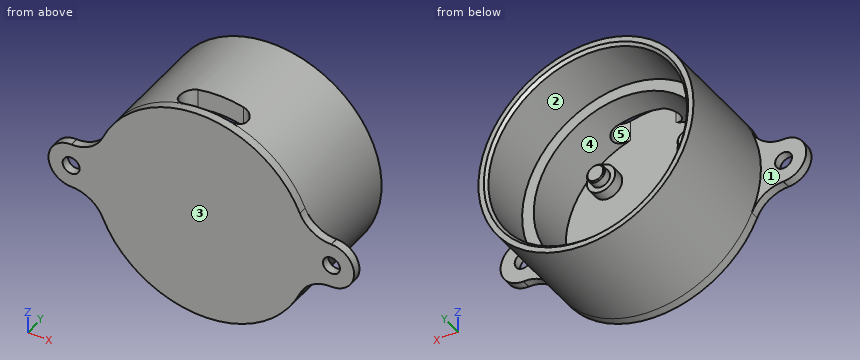
```python
from build123d import *

# Parameters (mm, degrees)
SKETCH_2_R               = 1.5
EXTRUDE_2_DEPTH          = 1.5
SKETCH_3_R               = 19
SKETCH_3_R_2             = 15.5
EXTRUDE_3_DEPTH          = 9
SKETCH_4_R               = 2.5
EXTRUDE_4_DEPTH          = 2
SKETCH_8_R               = 19
SKETCH_8_R_2             = 17.55
EXTRUDE_5_DEPTH          = 10
SKETCH_9_R               = 1.7
SKETCH_9_R_2             = 1.6
EXTRUDE_6_DEPTH          = 1.6
CUT_EXTRUDE_2_REACH      = 53.674
CUT_EXTRUDE_2_END_RADIUS = 15.5
CHAMFER_1_SIZE           = 0.5
CHAMFER_2_SIZE           = 0.2


with BuildPart() as part:
    # Эскиз2 → Бобышка-Вытянуть2 (new body)
    with BuildSketch(Plane(origin=(0, 0, 0), x_dir=(1, 0, 0), z_dir=(0, 1, 0))):
        with BuildLine():
            Line((-23, 4), (-22.912878475, 4))
            ThreePointArc((-22.912878475, 4), (-19.62654313, 4.980039841), (-17.413787641, 7.6))
            ThreePointArc((-17.413787641, 7.6), (0, 19), (17.413787641, 7.6))
            ThreePointArc((17.413787641, 7.6), (19.62654313, 4.980039841), (22.912878475, 4))
            Line((22.912878475, 4), (23, 4))
            ThreePointArc((23, 4), (27, 0), (23, -4))
            Line((23, -4), (22.912878475, -4))
            ThreePointArc((22.912878475, -4), (19.62654313, -4.980039841), (17.413787641, -7.6))
            ThreePointArc((17.413787641, -7.6), (0, -19), (-17.413787641, -7.6))
            ThreePointArc((-17.413787641, -7.6), (-19.62654313, -4.980039841), (-22.912878475, -4))
            Line((-22.912878475, -4), (-23, -4))
            ThreePointArc((-23, -4), (-27, 0), (-23, 4))
        make_face()
        with Locations(Location((-23, 0, 0), (0, 0, 270))):
            Circle(SKETCH_2_R, mode=Mode.SUBTRACT)
        with Locations(Location((23, 0, 0), (0, 0, 90))):
            Circle(SKETCH_2_R, mode=Mode.SUBTRACT)
    extrude(amount=EXTRUDE_2_DEPTH)

    # Эскиз3 → Бобышка-Вытянуть3 (add)
    with BuildSketch(Plane(origin=(0, 1.5, 0), x_dir=(1, 0, 0), z_dir=(0, 1, 0))):
        with Locations(Location((0, 0, 0), (0, 0, 23.578178478))):
            Circle(SKETCH_3_R)
        with Locations(Location((0, 0, 0), (0, 0, 270))):
            Circle(SKETCH_3_R_2, mode=Mode.SUBTRACT)
    extrude(amount=EXTRUDE_3_DEPTH)

    # Эскиз4 → Бобышка-Вытянуть4 (add)
    with BuildSketch(Plane(origin=(0, 1.5, 0), x_dir=(1, 0, 0), z_dir=(0, 1, 0))):
        with Locations(Location((-8, -8, 0), (0, 0, 90))):
            Circle(SKETCH_4_R)
        with Locations(Location((8, -8, 0), (0, 0, 90))):
            Circle(SKETCH_4_R)
        with Locations(Location((8, 8, 0), (0, 0, 90))):
            Circle(SKETCH_4_R)
        with Locations(Location((-8, 8, 0), (0, 0, 90))):
            Circle(SKETCH_4_R)
    extrude(amount=EXTRUDE_4_DEPTH)

    # Эскиз8 → Бобышка-Вытянуть5 (add)
    with BuildSketch(Plane(origin=(0, 10.5, 0), x_dir=(1, 0, 0), z_dir=(0, 1, 0))):
        with Locations(Location((0, 0, 0), (0, 0, 23.578178478))):
            Circle(SKETCH_8_R)
        with Locations(Location((0, 0, 0), (0, 0, 270))):
            Circle(SKETCH_8_R_2, mode=Mode.SUBTRACT)
    extrude(amount=EXTRUDE_5_DEPTH)

    # Эскиз9 → Бобышка-Вытянуть6 (add)
    with BuildSketch(Plane(origin=(0, 3.5, 0), x_dir=(1, 0, 0), z_dir=(0, 1, 0))):
        with Locations(Location((-8, 8, 0), (0, 0, 270))):
            Circle(SKETCH_9_R)
        with Locations(Location((8, 8, 0), (0, 0, 270))):
            Circle(SKETCH_9_R_2)
        with Locations(Location((-8, -8, 0), (0, 0, 270))):
            Circle(SKETCH_9_R_2)
        with Locations(Location((8, -8, 0), (0, 0, 270))):
            Circle(SKETCH_9_R_2)
    extrude(amount=EXTRUDE_6_DEPTH)

    # Вырез-Вытянуть2: up to this cylinder (the profile starts outside it)
    cut_extrude_2_end = Plane(origin=(0, 3.5, 0), z_dir=(0, -1, 0)) * Cylinder(CUT_EXTRUDE_2_END_RADIUS, 139.348, mode=Mode.PRIVATE)
    # Эскиз11 → Вырез-Вытянуть2 (cut, up to the surface)
    with BuildSketch(Plane.XY.offset(20), mode=Mode.PRIVATE) as cut_extrude_2_sk1:
        with BuildLine():
            Line((-4, 5.5), (4, 5.5))
            ThreePointArc((4, 5.5), (6, 3.5), (4, 1.5))
            Line((4, 1.5), (-4, 1.5))
            ThreePointArc((-4, 1.5), (-6, 3.5), (-4, 5.5))
        make_face()
    cut_extrude_2_tool1 = extrude(cut_extrude_2_sk1.sketch, amount=-CUT_EXTRUDE_2_REACH, mode=Mode.PRIVATE) - cut_extrude_2_end
    add(cut_extrude_2_tool1.solids().sort_by_distance((0, 3.5, 20))[0], mode=Mode.SUBTRACT)

    # Фаска1
    chamfer_1_edges = [part.edges().sort_by_distance(p)[0] for p in [
        (0, 20.5, -17.55),
    ]]
    chamfer(chamfer_1_edges, length=CHAMFER_1_SIZE)

    # Фаска2
    chamfer_2_edges = [part.edges().sort_by_distance(p)[0] for p in [
        (-8, 5.1, -9.7),
        (8, 5.1, -9.6),
        (-8, 5.1, 6.4),
        (8, 5.1, 6.4),
    ]]
    chamfer(chamfer_2_edges, length=CHAMFER_2_SIZE)


solid = part.part
```
Geometry check sheet. Reference: the model listing, model coordinates, mm. Face numbers are marked on the shaded views. A direction names the side the tool comes from. Give positions to 0.01 mm unless a question says otherwise; leave off trailing zeros. Write each loop counter-clockwise with the first axis right and the second up, starting at its lowest first coordinate (ties: lowest second). Pieces come first, ordered by that corner, then holes.
1) Section check B-B, the plane z = -0.5. State how many separate pieces and enclosed holes the cut face has, and give its area (3 significant figures).
2) Access from +Z, -Z, +X, -X, +Y, -Y to the whole of each face (thin tool, end or side, straight path). Record for the marked faces 3, 4 and 5.
3) Gauge pin test, flat ends, axial feed: pin 1 (1.4 mm diameter, centred on x = -7.5, z = 7.5, fed in from +Y); pin 2 (1.5 mm diameter, centred on x = 5, y = 16.5, fed in from -Z); pin 3 (4 mm diameter, centred on y = 16, z = 7.5, fed in from -X). Record the tip position at first contact, or that the pin passes through.
4) Release check for a two-part mould opening along X. For the marked faces 1 and 2 record: pulls with the +X half, pulls with the -X half, needs draft (parallel to the pull), parting line crosses it, or undercut.
5) Material ranges on L1, parallel to X at y = 1.15, z = 0; L2, parallel to X at y = 7, z = 0; L3, parallel to X at y = 14.25, z = 0, recorded low to high.
6) Section check A-A, the plane y = 2.5. Record the boundary of the cut face in (x, z).
Computed:
1. separate pieces: 3
1. enclosed holes: 0
1. area: 164 mm2
2. face 3: +Z, -Z, +X, -X, -Y
2. face 4: +Y
2. face 5: +Z
3. pin 1: stops at y = 5.1
3. pin 2: stops at z = -18.52
3. pin 3: stops at x = -18.19
4. face 1: needs draft
4. face 2: undercut
5. L1: x = -27 to -24.5, -21.5 to 21.5, 24.5 to 27
5. L2: x = -19 to -15.5, 15.5 to 19
5. L3: x = -19 to -17.55, 17.55 to 19
6. outline: circle Ø5 at (-8, -8); circle Ø5 at (-8, 8); (-5.73, 14.4) - (-5.73, 18.11) arc R19 ccw (long way) to (5.73, 18.11) - (5.73, 14.4) arc R15.5 cw (long way) to start; circle Ø5 at (8, -8); circle Ø5 at (8, 8)
